```python
from build123d import *

# Parameters (mm, degrees)
SKIZZE1_W                                            = 131
SKIZZE1_H                                            = 81
SKIZZE1_W_2                                          = 127
SKIZZE1_H_2                                          = 77
AUFSATZ_LINEAR_AUSTRAGEN1_DEPTH                      = 2
SKIZZE2_W                                            = 143
SKIZZE2_H                                            = 85
AUFSATZ_LINEAR_AUSTRAGEN2_DEPTH                      = 2
VERRUNDUNG1_R                                        = 3
FORMSENKUNG_F_R_M3_LINSENSENKSCHRAUBE_MI_D           = 3.4
FORMSENKUNG_F_R_M3_LINSENSENKSCHRAUBE_MI_DEPTH       = 7.25
FORMSENKUNG_F_R_M3_LINSENSENKSCHRAUBE_MI_CSINK_D     = 6.3
FORMSENKUNG_F_R_M3_LINSENSENKSCHRAUBE_MI_CSINK_ANGLE = 90
FORMSENKUNG_F_R_M3_LINSENSENKSCHRAUBE_MI_TIP         = 1.021463052


with BuildPart() as part:
    # Skizze1 → Aufsatz-Linear austragen1 (new body)
    with BuildSketch(Plane(origin=(0, 0, 0), x_dir=(1, 0, 0), z_dir=(0, 1, 0))):
        with Locations((65.5, 40.5)):
            Rectangle(SKIZZE1_W, SKIZZE1_H)
        with Locations((65.5, 40.5)):
            Rectangle(SKIZZE1_W_2, SKIZZE1_H_2, mode=Mode.SUBTRACT)
    extrude(amount=AUFSATZ_LINEAR_AUSTRAGEN1_DEPTH)

    # Skizze2 → Aufsatz-Linear austragen2 (add)
    with BuildSketch(Plane(origin=(0, 2, 0), x_dir=(1, 0, 0), z_dir=(0, 1, 0))):
        with Locations((65.5, 40.5)):
            Rectangle(SKIZZE2_W, SKIZZE2_H)
    extrude(amount=AUFSATZ_LINEAR_AUSTRAGEN2_DEPTH)

    # Verrundung1
    verrundung1_edges = [part.edges().sort_by_distance(p)[0] for p in [
        (-6, 3, -83),
        (-6, 3, 2),
        (137, 3, 2),
        (137, 3, -83),
        (0, 1, -81),
        (131, 1, -81),
        (131, 1, 0),
        (0, 1, 0),
    ]]
    fillet(verrundung1_edges, radius=VERRUNDUNG1_R)

    # Formsenkung für M3 Linsensenkschraube mit Schlitz1
    with Locations(Plane(origin=(0, 4, 0), x_dir=(1, 0, 0), z_dir=(0, 1, 0))):
        with Locations((-2, 2), (133, 79), (-2, 79), (133, 2)):
            CounterSinkHole(FORMSENKUNG_F_R_M3_LINSENSENKSCHRAUBE_MI_D / 2, FORMSENKUNG_F_R_M3_LINSENSENKSCHRAUBE_MI_CSINK_D / 2, depth=FORMSENKUNG_F_R_M3_LINSENSENKSCHRAUBE_MI_DEPTH, counter_sink_angle=FORMSENKUNG_F_R_M3_LINSENSENKSCHRAUBE_MI_CSINK_ANGLE)
            with Locations((0, 0, -(FORMSENKUNG_F_R_M3_LINSENSENKSCHRAUBE_MI_DEPTH + FORMSENKUNG_F_R_M3_LINSENSENKSCHRAUBE_MI_TIP / 2))):  # 118° drill point
                Cone(0, FORMSENKUNG_F_R_M3_LINSENSENKSCHRAUBE_MI_D / 2, FORMSENKUNG_F_R_M3_LINSENSENKSCHRAUBE_MI_TIP, mode=Mode.SUBTRACT)


solid = part.part
```
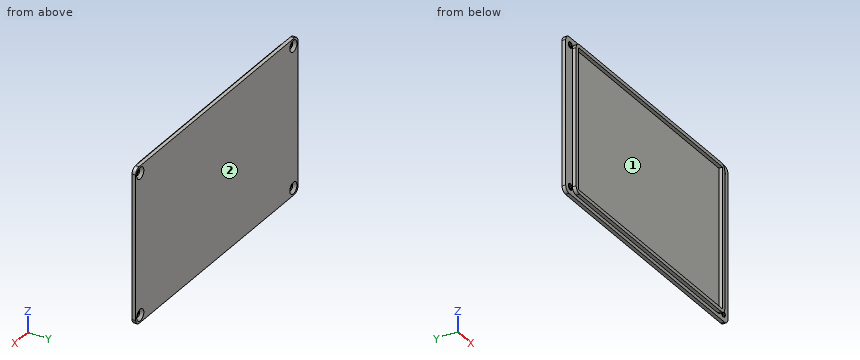
The listing builds one solid part. Answer for the finished solid, in the listing's coordinates (mm). Face numbers are marked on the shaded views. Round coordinates to 2 decimals unless told otherwise and drop trailing zeros. Write each loop counter-clockwise with the first axis right and the second up, starting at its lowest first coordinate (ties: lowest second). Pieces come first, ordered by that corner, then holes. Notation, with made-up numbers: (37, 2.5) -> (89, 2.5) arc R18 cw to (89, 18.5) -> close; hole circle Ø3 at (30.25, 34). An arc over 180 degrees is marked (long way). Answer as a JSON object with one key per item and string values. Group by question number.
Q1. Each of these flat-tipped pins is pushed along its axis until it touches: pin 1 Ø0.6 at (y, z) = (1, -55.5) entering from +X; pin 2 Ø5.5 at (x, z) = (-2, -2) entering from +Y; pin 3 Ø1 at (x, z) = (9.5, -48.5) entering from -Y. Where does it stop, or does it pass through?
Q2. Section B-B (z = -48) is taken. Write down the section's boundary in (x, y), plus the area to 3 significant figures.
Q3. Straight lines are drawn through the part: line 1 along X through (y, z) = (2.25, -79); line 2 along Z through (x, y) = (-2, 2.4); line 3 along X through (y, z) = (1.35, -66.5). For each, find the intervals that lie inside material, in ascending order.
Q4. Determine the mould class of the marked faces 1 and 2 for opening direction Z: pulls with the +Z half, pulls with the -Z half, needs draft (parallel to the pull), parting line crosses it, or undercut.
Q5. Section A-A (x = 39.5) is taken. Write down the section's boundary in (y, z).
Check values:
{
 "1": {"pin 1": "x = 131", "pin 2": "y = 3.6", "pin 3": "y = 2"},
 "2": {"outline": "(-6, 2) -> (0, 2) -> (0, 0) -> (2, 0) -> (2, 2) -> (129, 2) -> (129, 0) -> (131, 0) -> (131, 2) -> (137, 2) -> (137, 4) -> (-6, 4) -> close", "area": "294 mm^2"},
 "3": {"line 1": "-6 to -3.7, -0.3 to 131.3, 134.7 to 137", "line 2": "-83 to -80.7, -77.3 to -3.7, -0.3 to 2", "line 3": "0 to 2, 129 to 131"},
 "4": {"face 1": "undercut", "face 2": "needs draft"},
 "5": {"outline": "(0, -81) -> (2, -81) -> (2, -83) -> (4, -83) -> (4, 2) -> (2, 2) -> (2, 0) -> (0, 0) -> (0, -2) -> (2, -2) -> (2, -79) -> (0, -79) -> close"}
}
